Geometry: final body of the model. Coordinates: model frame, mm. Face numbers are marked on the shaded views. A direction names the side the tool comes from. Round coordinates to 2 decimals unless told otherwise and drop trailing zeros. Write each loop counter-clockwise with the first axis right and the second up, starting at its lowest first coordinate (ties: lowest second). Pieces come first, ordered by that corner, then holes.
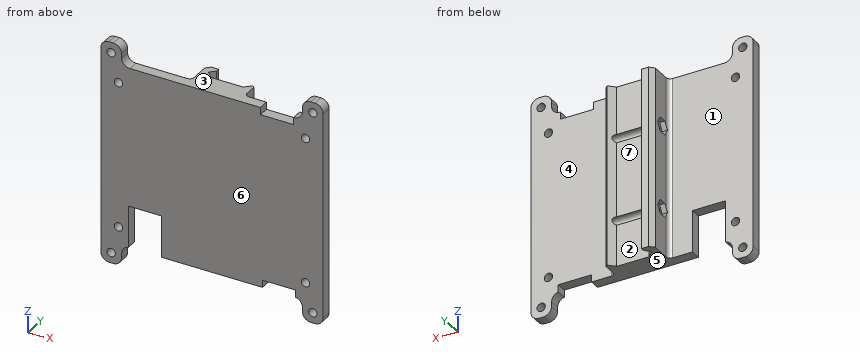
from build123d import *

# Parameters (mm, degrees)
BOSS_EXTRUDE1_DEPTH             = 87
CUT_EXTRUDE2_REACH              = 112.235
SKETCH7_R                       = 2.15
CUT_EXTRUDE3_DEPTH              = 2.5
F_4_0_START                     = -13.82
F_4_0_MM_DOWEL_HOLES1_OUTLINE_R = 2
F_4_0_MM_DOWEL_HOLES1_DEPTH     = 5.82
SKETCH11_W                      = 16
SKETCH11_H                      = 20.05000263
SKETCH11_H_2                    = 3.5
CUT_EXTRUDE4_DEPTH              = 10
SKETCH12_W                      = 10
SKETCH12_H                      = 10
SKETCH12_R                      = 2
BOSS_EXTRUDE2_DEPTH             = 5
MIRROR2_COPY_1_SKETCH_W         = 10
MIRROR2_COPY_1_SKETCH_H         = 10
MIRROR2_COPY_1_SKETCH_R         = 2
MIRROR2_COPY_1_DEPTH            = 5
FILLET1_R                       = 4
FILLET2_R                       = 2
CHAMFER1_SIZE                   = 2


with BuildPart() as part:
    # Sketch1 → Boss-Extrude1 (new body)
    with BuildSketch(Plane.XY):
        Polygon((0, 0), (2.5, 2.5), (2.5, 4.18), (-3, 4.18), (-3, -8.82), (-43.73, -8.82), (-43.73, -13.82), (63.27, -13.82), (63.27, -8.82), (22.54, -8.82), (22.54, -1.2), (21.54, -0.2), (18.61, -3.13), (3.13, -3.13), align=None)
    extrude(amount=BOSS_EXTRUDE1_DEPTH)

    # Sketch7 → Cut-Extrude2 (cut, up to next)
    with BuildSketch(Plane(origin=(22.54, 0, 0), x_dir=(0, 0, -1), z_dir=(1, 0, 0)), mode=Mode.PRIVATE) as cut_extrude2_sk1:
        with Locations(Location((-62, -3.82, 0), (0, 0, 90))):
            Circle(SKETCH7_R)
    cut_extrude2_tool1 = extrude(cut_extrude2_sk1.sketch, amount=-CUT_EXTRUDE2_REACH, mode=Mode.PRIVATE) & part.part
    # Sketch7 → Cut-Extrude2 (cut, up to next)
    with BuildSketch(Plane(origin=(22.54, 0, 0), x_dir=(0, 0, -1), z_dir=(1, 0, 0)), mode=Mode.PRIVATE) as cut_extrude2_sk2:
        with Locations(Location((-22, -3.82, 0), (0, 0, 90))):
            Circle(SKETCH7_R)
    cut_extrude2_tool2 = extrude(cut_extrude2_sk2.sketch, amount=-CUT_EXTRUDE2_REACH, mode=Mode.PRIVATE) & part.part
    add(cut_extrude2_tool1.solids().sort_by_distance((22.54, -3.82, 62))[0], mode=Mode.SUBTRACT)
    add(cut_extrude2_tool2.solids().sort_by_distance((22.54, -3.82, 22))[0], mode=Mode.SUBTRACT)

    # Sketch8 → Cut-Extrude3 (cut)
    with BuildSketch(Plane.ZY.offset(3)):
        Polygon((25.45, -5.811858429), (25.45, -1.828141571), (22, 0.163716857), (18.55, -1.828141571), (18.55, -5.811858429), (22, -7.803716857), align=None)
        Polygon((65.45, -5.811858429), (65.45, -1.828141571), (62, 0.163716857), (58.55, -1.828141571), (58.55, -5.811858429), (62, -7.803716857), align=None)
    extrude(amount=-CUT_EXTRUDE3_DEPTH, mode=Mode.SUBTRACT)

    # Ø4.0 mm Dowel Holes1: read off the stored shape, not the designer's step
    # Ø4.0 mm Dowel Holes1 outline → Ø4.0 mm Dowel Holes1 (cut)
    with BuildSketch(Plane(origin=(0, 0, 0), x_dir=(1, 0, 0), z_dir=(0, 1, 0)).offset(F_4_0_START)):
        with Locations((54.77, -78.5)):
            Circle(F_4_0_MM_DOWEL_HOLES1_OUTLINE_R)
        with Locations((-35.23, -8.5)):
            Circle(F_4_0_MM_DOWEL_HOLES1_OUTLINE_R)
        with Locations((54.77, -8.5)):
            Circle(F_4_0_MM_DOWEL_HOLES1_OUTLINE_R)
        with Locations((-35.23, -78.5)):
            Circle(F_4_0_MM_DOWEL_HOLES1_OUTLINE_R)
    extrude(amount=F_4_0_MM_DOWEL_HOLES1_DEPTH, mode=Mode.SUBTRACT)

    # Sketch11 → Cut-Extrude4 (cut)
    with BuildSketch(Plane.XZ.offset(13.82)):
        with Locations((-22.479997093, 10.025001315)):
            Rectangle(SKETCH11_W, SKETCH11_H)
        with Locations((42.054998939, 1.75)):
            Rectangle(SKETCH11_W, SKETCH11_H_2)
        with Locations((41.054998153, 85.25)):
            Rectangle(SKETCH11_W, SKETCH11_H_2)
    extrude(amount=-CUT_EXTRUDE4_DEPTH, mode=Mode.SUBTRACT)

    # Sketch12 → Boss-Extrude2 (add)
    with BuildSketch(Plane.XZ.offset(13.82)):
        with Locations((-38.73, -5)):
            Rectangle(SKETCH12_W, SKETCH12_H)
        with Locations(Location((-38.73, -5, 0), (0, 0, 270))):
            Circle(SKETCH12_R, mode=Mode.SUBTRACT)
    boss_extrude2 = extrude(amount=-BOSS_EXTRUDE2_DEPTH)

    # Mirror1: Boss-Extrude2 across plane
    add(boss_extrude2.mirror(Plane.XY.offset(43.5)))

    # Mirror2: Boss-Extrude2 across plane
    add(boss_extrude2.mirror(Plane.ZY.offset(-9.77)))

    # Mirror2 copy 1 sketch → Mirror2 copy 1 (add)
    with BuildSketch(Plane(origin=(19.54, -13.82, 87), x_dir=(-1, 0, 0), z_dir=(0, -1, 0))):
        with Locations((-38.73, -5)):
            Rectangle(MIRROR2_COPY_1_SKETCH_W, MIRROR2_COPY_1_SKETCH_H)
        with Locations(Location((-38.73, -5, 0), (0, 0, 270))):
            Circle(MIRROR2_COPY_1_SKETCH_R, mode=Mode.SUBTRACT)
    extrude(amount=-MIRROR2_COPY_1_DEPTH)

    # Fillet1
    # the kernel refuses this fillet: 4 mm, written as the material it adds along each edge
    with BuildSketch(Plane(origin=(-33.73, -13.82, 87), x_dir=(1, 0, 0), z_dir=(0, 1, 0)), Plane(origin=(53.27, -13.82, 87), x_dir=(0, 0, 1), z_dir=(0, 1, 0))) as fillet1_piece_1:
        with BuildLine():
            CenterArc((FILLET1_R, -FILLET1_R), FILLET1_R, 90, 90)
            Line((0, -FILLET1_R), (0, 0))
            Line((0, 0), (FILLET1_R, 0))
        make_face()
    extrude(amount=5)
    with BuildSketch(Plane(origin=(-33.73, -13.82, 0), x_dir=(1, 0, 0), z_dir=(0, 1, 0))) as fillet1_piece_2:
        with BuildLine():
            CenterArc((4, 3.929058966), FILLET1_R, 180, 79.193119511)
            Line((0, 3.929058966), (0, 0))
            Line((0, 0), (3.250002907, 0))
        make_face()
    extrude(amount=5)
    with BuildSketch(Plane(origin=(53.27, -13.82, 0), x_dir=(-1.0, -2.775557561562891e-15, -1.2049110107124816e-12), z_dir=(0, 1, 0))) as fillet1_piece_3:
        with BuildLine():
            CenterArc((4, -3.922215785), FILLET1_R, 101.317738871, 78.682261129)
            Line((0, -3.922215785), (0, 0))
            Line((0, 0), (3.215001061, 0))
        make_face()
    extrude(amount=5)
    # the kernel refuses this fillet: 4 mm, written as the material it takes off along each edge
    with BuildSketch(Plane(origin=(-33.73, -23.82, 97), x_dir=(-1, 0, 0), z_dir=(0, 1, 0)), Plane(origin=(-43.73, -23.82, 97), x_dir=(0, 0, -1), z_dir=(0, 1, 0)), Plane(origin=(-43.73, -23.82, -10), x_dir=(1, 0, 0), z_dir=(0, 1, 0)), Plane(origin=(-33.73, -23.82, -10), x_dir=(0, 0, 1), z_dir=(0, 1, 0))) as fillet1_2_piece_1:
        with BuildLine():
            CenterArc((FILLET1_R, -FILLET1_R), FILLET1_R, 90, 90)
            Line((0, -FILLET1_R), (0, 0))
            Line((0, 0), (FILLET1_R, 0))
        make_face()
    extrude(amount=25, mode=Mode.SUBTRACT)
    with BuildSketch(Plane(origin=(53.27, -23.82, -10), x_dir=(0, 0, 1), z_dir=(0, 1, 0)), Plane(origin=(53.27, -23.82, 97), x_dir=(1, 0, 0), z_dir=(0, 1, 0)), Plane(origin=(63.27, -23.82, 97), x_dir=(0, 0, -1), z_dir=(0, 1, 0)), Plane(origin=(63.27, -23.82, -10), x_dir=(-1, 0, 0), z_dir=(0, 1, 0))) as fillet1_2_piece_2:
        with BuildLine():
            CenterArc((FILLET1_R, FILLET1_R), FILLET1_R, 180, 90)
            Line((0, FILLET1_R), (0, 0))
            Line((0, 0), (FILLET1_R, 0))
        make_face()
    extrude(amount=25, mode=Mode.SUBTRACT)

    # Fillet2
    # the kernel refuses this fillet: 2 mm, written as the material it adds along each edge
    with BuildSketch(Plane(origin=(22.54, -8.82, 0), x_dir=(1, 0, 0), z_dir=(0, 0, 1))) as fillet2_piece_1:
        with BuildLine():
            CenterArc((FILLET2_R, FILLET2_R), FILLET2_R, 180, 90)
            Line((0, FILLET2_R), (0, 0))
            Line((0, 0), (FILLET2_R, 0))
        make_face()
    extrude(amount=87)
    with BuildSketch(Plane(origin=(-3, -8.82, 0), x_dir=(-1, 0, 0), z_dir=(0, 0, 1))) as fillet2_piece_2_section:
        with BuildLine():
            CenterArc((FILLET2_R, -FILLET2_R), FILLET2_R, 90, 90)
            Line((0, -FILLET2_R), (0, 0))
            Line((0, 0), (FILLET2_R, 0))
        make_face()
    fillet2_piece_2 = extrude(amount=87, mode=Mode.PRIVATE)
    fillet2_piece_2 = split(fillet2_piece_2, bisect_by=Plane(origin=(-3, -17.584067085, 5.059936491), z_dir=(0, 0.8660254037844386, -0.5000000000000001)), keep=Keep.TOP, mode=Mode.PRIVATE)
    fillet2_piece_2 = split(fillet2_piece_2, bisect_by=Plane(origin=(-3, 1.468491799, 5.940063509), z_dir=(0, -0.8660254037844385, -0.5000000000000003)), keep=Keep.TOP, mode=Mode.PRIVATE)
    add(fillet2_piece_2)
    with BuildSketch(Plane(origin=(-3, -8.82, 0), x_dir=(-1, 0, 0), z_dir=(0, 0, 1))) as fillet2_piece_3_section:
        with BuildLine():
            CenterArc((FILLET2_R, -FILLET2_R), FILLET2_R, 90, 90)
            Line((0, -FILLET2_R), (0, 0))
            Line((0, 0), (FILLET2_R, 0))
        make_face()
    fillet2_piece_3 = extrude(amount=87, mode=Mode.PRIVATE)
    fillet2_piece_3 = split(fillet2_piece_3, bisect_by=Plane(origin=(-3, -17.584067085, 5.059936491), z_dir=(0, -0.8660254037844386, 0.5000000000000001)), keep=Keep.TOP, mode=Mode.PRIVATE)
    fillet2_piece_3 = split(fillet2_piece_3, bisect_by=Plane(origin=(-3, 1.468491799, 5.940063509), z_dir=(0, -0.8660254037844385, -0.5000000000000003)), keep=Keep.TOP, mode=Mode.PRIVATE)
    add(fillet2_piece_3)
    with BuildSketch(Plane(origin=(-3, -8.82, 0), x_dir=(-1, 0, 0), z_dir=(0, 0, 1))) as fillet2_piece_4_section:
        with BuildLine():
            CenterArc((FILLET2_R, -FILLET2_R), FILLET2_R, 90, 90)
            Line((0, -FILLET2_R), (0, 0))
            Line((0, 0), (FILLET2_R, 0))
        make_face()
    fillet2_piece_4 = extrude(amount=87, mode=Mode.PRIVATE)
    fillet2_piece_4 = split(fillet2_piece_4, bisect_by=Plane(origin=(-3, -34.90457516, 15.059936491), z_dir=(0, 0.8660254037844385, -0.5000000000000003)), keep=Keep.TOP, mode=Mode.PRIVATE)
    fillet2_piece_4 = split(fillet2_piece_4, bisect_by=Plane(origin=(-3, 18.788999874, 15.940063509), z_dir=(0, -0.8660254037844385, -0.5000000000000003)), keep=Keep.TOP, mode=Mode.PRIVATE)
    fillet2_piece_4 = split(fillet2_piece_4, bisect_by=Plane(origin=(-3, -17.584067085, 5.059936491), z_dir=(0, -0.8660254037844386, 0.5000000000000001)), keep=Keep.TOP, mode=Mode.PRIVATE)
    fillet2_piece_4 = split(fillet2_piece_4, bisect_by=Plane(origin=(-3, 1.468491799, 5.940063509), z_dir=(0, 0.8660254037844385, 0.5000000000000003)), keep=Keep.TOP, mode=Mode.PRIVATE)
    add(fillet2_piece_4)
    with BuildSketch(Plane(origin=(-3, -8.82, 0), x_dir=(-1, 0, 0), z_dir=(0, 0, 1))) as fillet2_piece_5_section:
        with BuildLine():
            CenterArc((FILLET2_R, -FILLET2_R), FILLET2_R, 90, 90)
            Line((0, -FILLET2_R), (0, 0))
            Line((0, 0), (FILLET2_R, 0))
        make_face()
    fillet2_piece_5 = extrude(amount=87, mode=Mode.PRIVATE)
    fillet2_piece_5 = split(fillet2_piece_5, bisect_by=Plane(origin=(-3, -34.90457516, 15.059936491), z_dir=(0, -0.8660254037844385, 0.5000000000000003)), keep=Keep.TOP, mode=Mode.PRIVATE)
    fillet2_piece_5 = split(fillet2_piece_5, bisect_by=Plane(origin=(-3, 18.788999874, 15.940063509), z_dir=(0, -0.8660254037844385, -0.5000000000000003)), keep=Keep.TOP, mode=Mode.PRIVATE)
    add(fillet2_piece_5)
    with BuildSketch(Plane(origin=(-3, -8.82, 0), x_dir=(-1, 0, 0), z_dir=(0, 0, 1))) as fillet2_piece_6_section:
        with BuildLine():
            CenterArc((FILLET2_R, -FILLET2_R), FILLET2_R, 90, 90)
            Line((0, -FILLET2_R), (0, 0))
            Line((0, 0), (FILLET2_R, 0))
        make_face()
    fillet2_piece_6 = extrude(amount=87, mode=Mode.PRIVATE)
    fillet2_piece_6 = split(fillet2_piece_6, bisect_by=Plane(origin=(-3, -34.90457516, 15.059936491), z_dir=(0, -0.8660254037844385, 0.5000000000000003)), keep=Keep.TOP, mode=Mode.PRIVATE)
    fillet2_piece_6 = split(fillet2_piece_6, bisect_by=Plane(origin=(-3, 18.788999874, 15.940063509), z_dir=(0, 0.8660254037844385, 0.5000000000000003)), keep=Keep.TOP, mode=Mode.PRIVATE)
    add(fillet2_piece_6)

    # Chamfer1
    chamfer1_edges = [part.edges().sort_by_distance(p)[0] for p in [
        (-3, 4.18, 43.5),
    ]]
    chamfer(chamfer1_edges, length=CHAMFER1_SIZE)


solid = part.part
1) Section A-A on z = 8.5. State how many separate pieces and enclosed holes the cut face has, plus the area to 3 significant figures.
2) Reachability of the marked faces 1, 2, 3, 4 and 5 from +Z, -Z, +X, -X, +Y, -Y: full face, straight path, thin tool, end or side. Return the list, or none.
3) First-contact query: P1, Ø1, axis at y = -5.5, z = 78, coming from the +X side; P2, Ø7.5, axis at x = 12.5, z = 43.5, coming from the +Y side; P3, Ø5.5, axis at y = -3, z = 22.5, coming from the -X side. Flat tips, straight axial feed; report the tip coordinate or a pass-through.
4) Draft query along X for the marked faces 6 and 7. Return one class per face: pulls with the +X half, pulls with the -X half, needs draft (parallel to the pull), parting line crosses it, or undercut.
5) Section B-B on x = 15. Output: boundary loops of the cut face in (y, z).
6) Section C-C on x = -35.23. Output: boundary loops of the cut face in (y, z).
7) Line query: probe 1 along Z at (x, y) = (58.27, -10.55); probe 2 along Z at (x, y) = (10.5, -3.82); probe 3 along X at (y, z) = (-11.25, 78.5). Output: solid intervals per line, ascending.
Filled in:
1. separate pieces: 4
1. enclosed holes: 0
1. area: 601 mm2
2. face 1: +Z, -Z, -X, +Y
2. face 2: +Z, -Z, +Y
2. face 3: +Z, +Y, -Y
2. face 4: +Z, -Z, +X, +Y
2. face 5: -Z, +Y, -Y
3. P1: stops at x = 22.54
3. P2: stops at y = -3.13
3. P3: stops at x = -3
4. face 6: needs draft
4. face 7: undercut
5. outline: (-13.82, 0) - (-3.13, 0) - (-3.13, 19.96) arc R2.15 cw (long way) to (-3.13, 24.04) - (-3.13, 59.96) arc R2.15 cw (long way) to (-3.13, 64.04) - (-3.13, 87) - (-13.82, 87) - close
6. outline: (-13.82, -9.12) - (-8.82, -9.12) - (-8.82, 6.5) - (-13.82, 6.5) - close; (-13.82, 10.5) - (-8.82, 10.5) - (-8.82, 76.5) - (-13.82, 76.5) - close; (-13.82, 80.5) - (-8.82, 80.5) - (-8.82, 96.12) - (-13.82, 96.12) - close
7. probe 1: z = -10 to -7, -3 to 90, 94 to 97
7. probe 2: z = 0 to 19.85, 24.15 to 59.85, 64.15 to 87
7. probe 3: x = -43.73 to -37.23, -33.23 to 52.77, 56.77 to 63.27
